```python
from build123d import *

# Parameters (mm, degrees)
F0_W     = 123.919994
F0_H     = 59.413508
F0_R     = 6.14177
F1_DEPTH = 25


with BuildPart() as f1:
    # F0 (on Top) → F1 (new body)
    with BuildSketch(Plane.XY):
        Rectangle(F0_W, F0_H)
        Polygon((-42.643782, 6.749166), (-42.643782, 18.240707), (-29.568307, 18.240707), (-29.568307, 12.494937), (-29.568307, 6.749166), align=None, mode=Mode.SUBTRACT)
        Circle(F0_R, mode=Mode.SUBTRACT)
    extrude(amount=F1_DEPTH)


solid = f1.part
```
Source: CAD feature listing. Evaluate the final solid. Frame: model axes, mm. A direction names the side the tool comes from. Round coordinates to 2 decimals unless told otherwise and drop trailing zeros. Loops run counter-clockwise (first coordinate to the right, second up) from the corner with the lowest first, then second, coordinate; pieces in that order, holes last.
(1) Pull-direction query (X, two-part tool) for faces 3 (the flat face through (61.96, 0, 12)), 4 (the flat face through (-61.96, 0, 12)), 5 (the flat face through (-36, 18.241, 12)), 6 (the flat face through (-1, 29.707, 12)); classes: +X half, -X half, draft (parallel to the pull), parting line (faces both ways), or undercut.
From the geometry:
face 3: +X half
face 4: -X half
face 5: undercut
face 6: draft
(2) Section query C-C (y = 0). Output: boundary loops of the cut face in (x, z).
From the geometry:
outline: (-61.96, 0) - (-6.14, 0) - (-6.14, 25) - (-61.96, 25) - close; (6.14, 0) - (61.96, 0) - (61.96, 25) - (6.14, 25) - close
(3) Material intervals for probe 1 along X at (y, z) = (14, 9.75); probe 2 along Y at (x, z) = (0, 17.5); probe 3 along Y at (x, z) = (-2, 2.75), sorted ascending.
From the geometry:
probe 1: x = -61.96 to -42.64, -29.57 to 61.96
probe 2: y = -29.71 to -6.14, 6.14 to 29.71
probe 3: y = -29.71 to -5.81, 5.81 to 29.71
(4) Contact query for a flat-ended pin moving along its axis: pin 1 Ø10 at (x, y) = (-42.5, 8) entering from -Z. Output: stop coordinate, or through.
From the geometry:
pin 1: stops at z = 0
(5) Access query for faces 1 (the flat face through (-1, -29.707, 12)), 2 (the flat face through (-36, 6.749, 12)). Directions: +Z, -Z, +X, -X, +Y, -Y. A direction counts if a zero-diameter tool reaches every point of the face in a straight line with its end or side. Return the directions, or none.
From the geometry:
face 1: +Z, -Z, +X, -X, -Y
face 2: +Z, -Z
(6) Section query B-B (z = 3.25). Output: boundary loops of the cut face in (x, y), and give its area (3 significant figures).
From the geometry:
outline: (-61.96, -29.71) - (61.96, -29.71) - (61.96, 29.71) - (-61.96, 29.71) - close; hole (-42.64, 6.75) - (-29.57, 6.75) - (-29.57, 18.24) - (-42.64, 18.24) - close; hole circle Ø12.28 at (0, 0)
area: 7,090 mm2
(7) Section query A-A (x = 0). Output: boundary loops of the cut face in (y, z).
From the geometry:
outline: (-29.71, 0) - (-6.14, 0) - (-6.14, 25) - (-29.71, 25) - close; (6.14, 0) - (29.71, 0) - (29.71, 25) - (6.14, 25) - close
